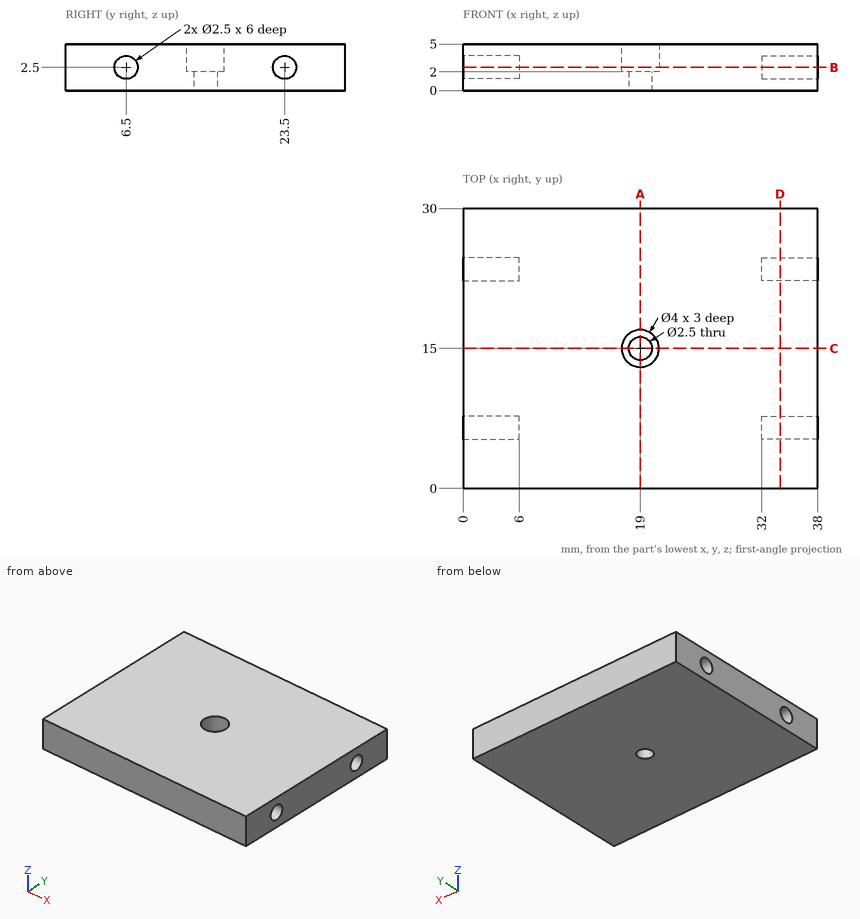
Job drawing, mm, ordinate dimensions from the low corner. One solid piece. Round coordinates to 2 decimals unless told otherwise and drop trailing zeros. Loops run counter-clockwise (first coordinate to the right, second up) from the corner with the lowest first, then second, coordinate; pieces in that order, holes last. Notation, with made-up numbers: (-22.5, 2) -> (32.5, 2) arc R23 ccw to (32.5, 39) -> close; hole circle Ø7 at (29.25, 87.5). An arc over 180 degrees is marked (long way). One line per item, written item: value. Start each with the question number.
Q1. Probe line 1 along Y through (x, z) = (5.5, 1.55); line 2 along Z through (x, y) = (36, 23.5); line 3 along Y through (x, z) = (19, 3.35). List the from-to ranges inside material, lowest first.
Q2. Cut at A-A on x = 19. List the corners of the cut face in (y, z), plus the area to 3 significant figures.
Q3. Cut at D-D on x = 34. List the corners of the cut face in (y, z), plus the area to 3 significant figures.
Q4. Cut at B-B on z = 2.5. List the corners of the cut face in (x, y).
Q5. Drop flat-ended pins along their axis: pin 1 Ø1.5 at (y, z) = (23.5, 2.5) entering from -X; pin 2 Ø1.2 at (y, z) = (6.5, 2.5) entering from +X; pin 3 Ø3 at (x, y) = (19, 15) entering from +Z. Give the stop position or say it passes through.
Q6. Cut at C-C on y = 15. List the corners of the cut face in (x, z), plus the area to 3 significant figures.
Computed:
1. line 1: 0 to 5.69, 7.31 to 22.69, 24.31 to 30
1. line 2: 0 to 1.25, 3.75 to 5
1. line 3: 0 to 13, 17 to 30
2. outline: (0, 0) -> (13.75, 0) -> (13.75, 2) -> (13, 2) -> (13, 5) -> (0, 5) -> close; (16.25, 0) -> (30, 0) -> (30, 5) -> (17, 5) -> (17, 2) -> (16.25, 2) -> close
2. area: 133 mm²
3. outline: (0, 0) -> (30, 0) -> (30, 5) -> (0, 5) -> close; hole circle Ø2.5 at (6.5, 2.5); hole circle Ø2.5 at (23.5, 2.5)
3. area: 140 mm²
4. outline: (0, 0) -> (38, 0) -> (38, 5.25) -> (32, 5.25) -> (32, 7.75) -> (38, 7.75) -> (38, 22.25) -> (32, 22.25) -> (32, 24.75) -> (38, 24.75) -> (38, 30) -> (0, 30) -> (0, 24.75) -> (6, 24.75) -> (6, 22.25) -> (0, 22.25) -> (0, 7.75) -> (6, 7.75) -> (6, 5.25) -> (0, 5.25) -> close; hole circle Ø4 at (19, 15)
5. pin 1: x = 6
5. pin 2: x = 32
5. pin 3: z = 2
6. outline: (0, 0) -> (17.75, 0) -> (17.75, 2) -> (17, 2) -> (17, 5) -> (0, 5) -> close; (20.25, 0) -> (38, 0) -> (38, 5) -> (21, 5) -> (21, 2) -> (20.25, 2) -> close
6. area: 173 mm²
